Input: part model. Units: mm. Frame: model coordinates. A direction names the side the tool comes from. Coordinates: 2 decimals unless noted, no trailing zeros. Order: outer loops, then holes, each group sorted by start corner. A loop starts at its lowest first (then second) coordinate and runs counter-clockwise, first axis right, second up. Notation, with made-up numbers: M -0.75,37.5 L 7.25,37.5 A20 cw 7.25,71.5 Z; hole C 87.5,-29.5 d3. An arc over 180 degrees is marked long. One line per item, written item: value.
```python
from build123d import *

# Parameters (mm, degrees)
SKETCH_1_R      = 85
SKETCH_1_R_2    = 70
EXTRUDE_1_DEPTH = 14
SHELL_1_T       = -2


with BuildPart() as part:
    # 草图1 → 凸台-拉伸1 (new body)
    with BuildSketch(Plane.XY):
        Circle(SKETCH_1_R)
        Circle(SKETCH_1_R_2, mode=Mode.SUBTRACT)
    extrude(amount=EXTRUDE_1_DEPTH)

    # 抽壳1
    shell_1_openings = [part.faces().sort_by_distance(p)[0] for p in [
        (-82.595836944, 0, 14),
    ]]
    offset(amount=SHELL_1_T, openings=shell_1_openings, kind=Kind.INTERSECTION)


solid = part.part
```
(1) Cut plane A-A on y = 0. Output: boundary loops of the cut face in (x, z), plus the area to 3 significant figures.
Data:
outline: M -85,0 L -70,0 L -70,14 L -72,14 L -72,2 L -83,2 L -83,14 L -85,14 Z; M 70,0 L 85,0 L 85,14 L 83,14 L 83,2 L 72,2 L 72,14 L 70,14 Z
area: 156 mm2
(2) Ray query, line 1 (Y direction, x = 0, z = 7.5); line 2 (Y direction, x = 2.5, z = 6.75). Return the intervals inside material, ascending. Write a range as from..to.
Data:
line 1: y = -85..-83, -72..-70, 70..72, 83..85
line 2: y = -84.96..-82.96, -71.96..-69.96, 69.96..71.96, 82.96..84.96
(3) Cut plane D-D on x = -74. Output: boundary loops of the cut face in (y, z), plus the area to 3 significant figures.
Data:
outline: M -41.82,0 L 41.82,0 L 41.82,14 L 37.59,14 L 37.59,2 L -37.59,2 L -37.59,14 L -41.82,14 Z
area: 269 mm2
(4) Cut plane C-C on z = 9.5. Output: boundary loops of the cut face in (x, y).
Data:
outline: C 0,0 d170; C 0,0 d144; hole C 0,0 d166; hole C 0,0 d140
(5) Draft query along Y for faces 1 (the cylindrical face through (-9.373, 71.387, 7.916)), 2 (the cylindrical face through (-67.453, -51.721, 6.902)), 3 (the flat face through (18.5, -81.5, 14)). Return one class per face: released by +Y, released by -Y, zero draft, split by the parting line, or undercut.
Data:
face 1: undercut
face 2: split by the parting line
face 3: zero draft
(6) Access query for faces 4 (the flat face through (-59, 38, 14)), 5 (the flat face through (-25, 68, 2)). Directions: +Z, -Z, +X, -X, +Y, -Y. A direction counts if a zero-diameter tool reaches every point of the face in a straight line with its end or side. Return the directions, or none.
Data:
face 4: +Z, +X, -X, +Y, -Y
face 5: +Z
(7) First-contact query: pin 1 (5 mm diameter, centred on x = 5.5, z = 6, fed in from +Y); pin 2 (1.5 mm diameter, centred on x = 50.5, z = 7, fed in from +Y); pin 3 (6 mm diameter, centred on x = 49, y = 55.5, fed in from +Z); pin 4 (1.5 mm diameter, centred on x = 34.5, z = 10, fed in from -Y). Flat tips, straight axial feed; report the tip coordinate or a pass-through.
Data:
pin 1: stops at y = 84.95
pin 2: stops at y = 68.92
pin 3: stops at z = 14
pin 4: stops at y = -78.01
